Here's how the part is built. I have some questions about the finished solid (model axes, mm). A direction names the side the tool comes from. Round coordinates to 2 decimals unless told otherwise and drop trailing zeros. Write each loop counter-clockwise with the first axis right and the second up, starting at its lowest first coordinate (ties: lowest second). Pieces come first, ordered by that corner, then holes. Notation, with made-up numbers: (-11, -22) -> (4, -22) arc R29 cw to (4, 6) -> close; hole circle Ø7 at (7.5, -3.5). An arc over 180 degrees is marked (long way). Answer as CSV lines item,"result".
from build123d import *

# Parameters (mm, degrees)
F0_W     = 5
F0_H     = 66
F0_W_2   = 16.5
F0_W_3   = 65
F1_DEPTH = 21
F2_DEPTH = 4
F3_W     = 108
F3_H     = 2
F4_DEPTH = 8


with BuildPart() as f1:
    # F0 (on Front) → F1 (new body)
    with BuildSketch(Plane.XZ):
        with Locations((-35, -33)):
            Rectangle(F0_W, F0_H)
        with Locations((-45.75, -33)):
            Rectangle(F0_W_2, F0_H)
        with Locations((0, -33)):
            Rectangle(F0_W_3, F0_H)
        with Locations((35, -33)):
            Rectangle(F0_W, F0_H)
        with Locations((45.75, -33)):
            Rectangle(F0_W_2, F0_H)
    extrude(amount=F1_DEPTH)

    # F0 (on Front) → F2 (join)
    with BuildSketch(Plane.XZ):
        with Locations((35, -33)):
            Rectangle(F0_W, F0_H)
        with Locations((-35, -33)):
            Rectangle(F0_W, F0_H)
    extrude(amount=-F2_DEPTH)

    # F3 (on face) → F4 (join)
    with BuildSketch(Plane.XZ.offset(21)):
        with Locations((0, -1)):
            Rectangle(F3_W, F3_H)
    extrude(amount=F4_DEPTH)


solid = f1.part
Item 1: Suppose I cut it at B-B, the plane z = -58.5. List the corners of the cut face in (x, y) for me, then the cut area to 3 significant figures.
Results found:
outline,"(-54, -21) -> (54, -21) -> (54, 0) -> (37.5, 0) -> (37.5, 4) -> (32.5, 4) -> (32.5, 0) -> (-32.5, 0) -> (-32.5, 4) -> (-37.5, 4) -> (-37.5, 0) -> (-54, 0) -> close"
area,"2,310 mm²"
Item 2: For faces 1 (the flat face through (-46, 0, -33)), 2 (the flat face through (0, 0, -33)), 3 (the flat face through (-1, -21, -34)), 4 (the flat face through (46, 0, -33)), which set-ups out of +Z, -Z, +X, -X, +Y, -Y let a thin tool reach every point of the face, with its end or its side?
Results found:
face 1,"+Z, -Z, -X, +Y"
face 2,"+Z, -Z, +Y"
face 3,"-Z, +X, -X, -Y"
face 4,"+Z, -Z, +X, +Y"
Item 3: If we mould it in two halves opening along X, with no side actions, what happens to faces 5 (the flat face through (32.5, 2, -33)), 6 (the flat face through (-37.5, 2, -33)), 7 (the flat face through (-1, -11, -66)), 8 (the flat face through (37.5, 2, -33))? For each: pulls with the +X half, pulls with the -X half, needs draft (parallel to the pull), parting line crosses it, or undercut.
Results found:
face 5,"undercut"
face 6,"pulls with the -X half"
face 7,"needs draft"
face 8,"pulls with the +X half"
Item 4: Will these pins go through, and if not, where does the flat tip stop? pin 1 (19.5 mm diameter, centred on x = -2, z = -33.5, fed in from +Y); pin 2 (3 mm diameter, centred on y = 2, z = -17.5, fed in from -X); pin 3 (3 mm diameter, centred on y = 2.5, z = -49, fed in from +X).
Results found:
pin 1,"stops at y = 0"
pin 2,"stops at x = -37.5"
pin 3,"stops at x = 37.5"
Item 5: I need wall thicknesses on L1, parallel to Z at x = 8, y = -25; L2, parallel to Y at x = -34, z = -60.5; L3, parallel to Y at x = 17.5, z = -9.5. Which ranges of each line are inside material? Lowest first, please.
Results found:
L1,"z = -2 to 0"
L2,"y = -21 to 4"
L3,"y = -21 to 0"
Item 6: Suppose I cut it at A-A, the plane x = -34. List the corners of the cut face in (y, z) for me.
Results found:
outline,"(-29, -2) -> (-21, -2) -> (-21, -66) -> (4, -66) -> (4, 0) -> (-29, 0) -> close"
Item 7: Suppose I cut it at C-C, the plane y = -23. List the corners of the cut face in (x, z) for me.
Results found:
outline,"(-54, -2) -> (54, -2) -> (54, 0) -> (-54, 0) -> close"
